Here's how the part is built. I have some questions about the finished solid (model axes, mm). A direction names the side the tool comes from. Coordinates: 2 decimals unless noted, no trailing zeros. Write each loop counter-clockwise with the first axis right and the second up, starting at its lowest first coordinate (ties: lowest second). Pieces come first, ordered by that corner, then holes.
from build123d import *

# Parameters (mm, degrees)
SKIZZE1_W                       = 20
SKIZZE1_H                       = 33.6
AUFSATZ_LINEAR_AUSTRAGEN1_DEPTH = 3
SKIZZE3_W                       = 171.2
SKIZZE3_H                       = 6.4
AUFSATZ_LINEAR_AUSTRAGEN2_DEPTH = 7


with BuildPart() as part:
    # Skizze1 → Aufsatz-Linear austragen1 (new body)
    with BuildSketch(Plane(origin=(0, 0, 0), x_dir=(1, 0, 0), z_dir=(0, 1, 0))):
        with Locations((10, 23.2)):
            Rectangle(SKIZZE1_W, SKIZZE1_H)
        Polygon((0, 6.4), (0, 0), (171.2, 0), (171.2, 40), (151.2, 40), (151.2, 6.4), (133.4, 6.4), (133.4, 40), (113.4, 40), (113.4, 6.4), (95.6, 6.4), (95.6, 40), (75.6, 40), (75.6, 6.4), (57.8, 6.4), (57.8, 40), (37.8, 40), (37.8, 6.4), (20, 6.4), align=None)
    extrude(amount=AUFSATZ_LINEAR_AUSTRAGEN1_DEPTH)

    # Skizze3 → Aufsatz-Linear austragen2 (add)
    with BuildSketch(Plane(origin=(0, 3, 0), x_dir=(1, 0, 0), z_dir=(0, 1, 0))):
        with Locations((85.6, 3.2)):
            Rectangle(SKIZZE3_W, SKIZZE3_H)
    extrude(amount=AUFSATZ_LINEAR_AUSTRAGEN2_DEPTH)


solid = part.part
1. For pin 1 Ø22 at (x, z) = (44, -25) entering from +Y, with a flat end and sliding along its axis, tell me the tip position at first contact or that it passes through.
2. Thinking about a two-plate mould opening in X: for faces 1 (the face through (48, 1, -40)), 2 (the face through (0, 2.7, -15.3)), 3 (the face through (133.4, 1, -23)), which applies, pulls with the +X half, pulls with the -X half, needs draft (parallel to the pull), parting line crosses it, or undercut?
3. I want a section at B-B (x = 90). List the corners of the cut face in (y, z) for me, then the cut area to 3 significant figures.
4. I want a section at A-A (z = -14). List the corners of the cut face in (x, y) for me, then the cut area to 3 significant figures.
5. I want a section at D-D (x = 110). List the corners of the cut face in (y, z) for me.
6. I want a section at C-C (y = 6.5). List the corners of the cut face in (x, z) for me.
7. On a 3-axis mill with a long thin cutter (end or side, diameter ignored), from which of +Z, -Z, +X, -X, +Y, -Y can I reach the whole of each face in a straight line? I mean faces 4 (the face through (37.8, 1, -23)), 5 (the face through (84, 10, -3)), 6 (the face through (10, 3, -23)). Say none if no direction works.
8. If I drill on line 1 (X direction, y = 2.5, z = -22); line 2 (Z direction, x = 54.5, y = 5); line 3 (Y direction, x = 92, z = -27.5), over which ranges is the centre line in solid material (lowest first)?
Response values:
1. pin 1: stops at y = 3
2. face 1: needs draft
2. face 2: pulls with the -X half
2. face 3: undercut
3. outline: (0, -40) - (3, -40) - (3, -6.4) - (10, -6.4) - (10, 0) - (0, 0) - close
3. area: 165 mm2
4. outline: (0, 0) - (20, 0) - (20, 3) - (0, 3) - close; (37.8, 0) - (57.8, 0) - (57.8, 3) - (37.8, 3) - close; (75.6, 0) - (95.6, 0) - (95.6, 3) - (75.6, 3) - close; (113.4, 0) - (133.4, 0) - (133.4, 3) - (113.4, 3) - close; (151.2, 0) - (171.2, 0) - (171.2, 3) - (151.2, 3) - close
4. area: 300 mm2
5. outline: (0, -6.4) - (10, -6.4) - (10, 0) - (0, 0) - close
6. outline: (0, -6.4) - (171.2, -6.4) - (171.2, 0) - (0, 0) - close
7. face 4: -Z, +Y, -Y
7. face 5: +Z, -Z, +X, -X, +Y
7. face 6: -Z, +X, -X, +Y
8. line 1: x = 0 to 20, 37.8 to 57.8, 75.6 to 95.6, 113.4 to 133.4, 151.2 to 171.2
8. line 2: z = -6.4 to 0
8. line 3: y = 0 to 3
